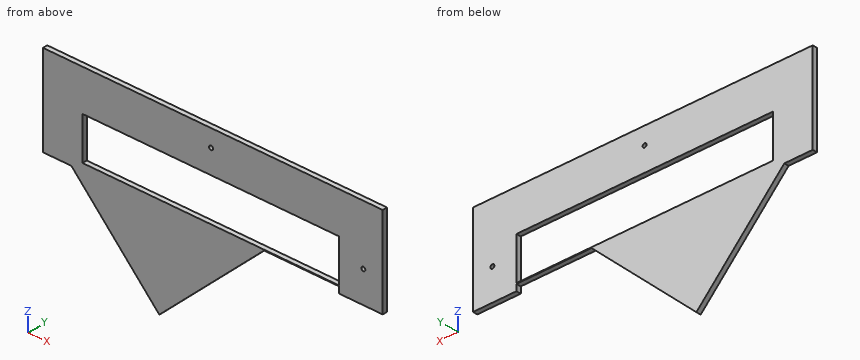
```python
from build123d import *

# Parameters (mm, degrees)
F0_W     = 325
F0_H     = 54
F0_R     = 2.5
F1_DEPTH = 6


# Not quite as in the source:
# - a feature names something its author has since deleted; it is built from what else it names


with BuildPart() as f1:
    # F0 (on Front) → F1 (new body)
    with BuildSketch(Plane.XZ):
        Polygon((0, 115), (0, 0), (35.9275913919, 0), (50, 0), (50, 8), (279.8869819123, 8), (375, 8), (375, 0), (430, 0), (430, 115), align=None)
        with Locations((212.5, 36)):
            Rectangle(F0_W, F0_H, mode=Mode.SUBTRACT)
        with Locations((212.7146603412, 93.1771022268)):
            Circle(F0_R, mode=Mode.SUBTRACT)
        with Locations((405.4770870114, 39.8606238714)):
            Circle(F0_R, mode=Mode.SUBTRACT)
        Polygon((50, 0), (35.9275913919, 0), (147.2313553095, -117.5774261355), (279.8869819123, 8), (50, 8), align=None)
    extrude(amount=F1_DEPTH)


solid = f1.part
```
Could you check a few things on this model? Use its own coordinates, in mm. Coordinates: 2 decimals unless noted, no trailing zeros. Write each loop counter-clockwise with the first axis right and the second up, starting at its lowest first coordinate (ties: lowest second). Pieces come first, ordered by that corner, then holes. Notation, with made-up numbers: (52.5, 39) -> (73.5, 39) arc R14 cw to (73.5, 57) -> close; hole circle Ø5 at (-3, 67.5). An arc over 180 degrees is marked (long way). One line per question, with ' | ' between items. Start each with the question number.
1. Will these pins go through, and if not, where does the flat tip stop? P1, Ø8, axis at x = 212.71, z = 93.18, coming from the -Y side; P2, Ø3, axis at x = 405, y = -1.5, coming from the -Z side.
2. Please list where these lines run through material, in increasing order: line 1 along X through (y, z) = (-3.7, 40); line 2 along Z through (x, y) = (352, -0.8); line 3 along X through (y, z) = (-3.9, 11.5).
3. If we section it at B-B (x = 293): Please give me the cut outline in (y, z), and give its area (3 significant figures).
4. If we section it at D-D (z = -90.5): Please give me the cut outline in (x, y) (3 decimals).
5. If we section it at C-C (y = -2.65): Please give me the cut outline in (x, z), and give its area (3 significant figures).
6. If we section it at A-A (z = 59): Please give me the cut outline in (x, y), and give its area (3 significant figures).
Return value:
1) P1: stops at y = -6 | P2: stops at z = 0
2) line 1: x = 0 to 50, 375 to 402.98, 407.97 to 430 | line 2: z = 8 to 9, 63 to 115 | line 3: x = 0 to 50, 375 to 430
3) outline: (-6, 8) -> (0, 8) -> (0, 9) -> (-6, 9) -> close; (-6, 63) -> (0, 63) -> (0, 115) -> (-6, 115) -> close | area: 318 mm²
4) outline: (121.599, -6) -> (175.835, -6) -> (175.835, 0) -> (121.599, 0) -> close
5) outline: (0, 0) -> (35.93, 0) -> (147.23, -117.58) -> (279.89, 8) -> (375, 8) -> (375, 0) -> (430, 0) -> (430, 115) -> (0, 115) -> close; hole (50, 9) -> (375, 9) -> (375, 63) -> (50, 63) -> close; hole circle Ø5 at (212.71, 93.18); hole circle Ø5 at (405.48, 39.86) | area: 44,900 mm²
6) outline: (0, -6) -> (50, -6) -> (50, 0) -> (0, 0) -> close; (375, -6) -> (430, -6) -> (430, 0) -> (375, 0) -> close | area: 630 mm²
